Input: dimensioned drawing with shaded views. Units: mm. Origin: part minimum x, y, z. A direction names the side the tool comes from. Coordinates: 2 decimals unless noted, no trailing zeros. Loops run counter-clockwise (first coordinate to the right, second up) from the corner with the lowest first, then second, coordinate; pieces in that order, holes last.
Item 1: Section query B-B, the plane y = 1. Return the cut outline in (x, z).
Item 2: Reachability of the marked faces 1, 2, 3 and 4 from +Z, -Z, +X, -X, +Y, -Y: full face, straight path, thin tool, end or side. Return the list, or none.
Item 3: Line query: probe 1 along X at (y, z) = (5, 1.5); probe 2 along Z at (x, y) = (1.75, 4.25); probe 3 along Z at (x, y) = (5.75, 9.25). Output: solid intervals per line, ascending.
Item 4: Section query A-A, the plane z = 9.5. Return the cut outline in (x, y).
Item 5: Pin query (flat end, axial travel): pin 1 Ø1 at (x, z) = (3.5, 7.5) entering from +Y; pin 2 Ø1.5 at (x, z) = (2, 5.5) entering from -Y; pin 3 Ø1 at (y, z) = (1, 7) entering from -X. Return the tip coordinate at first contact, or that it passes through.
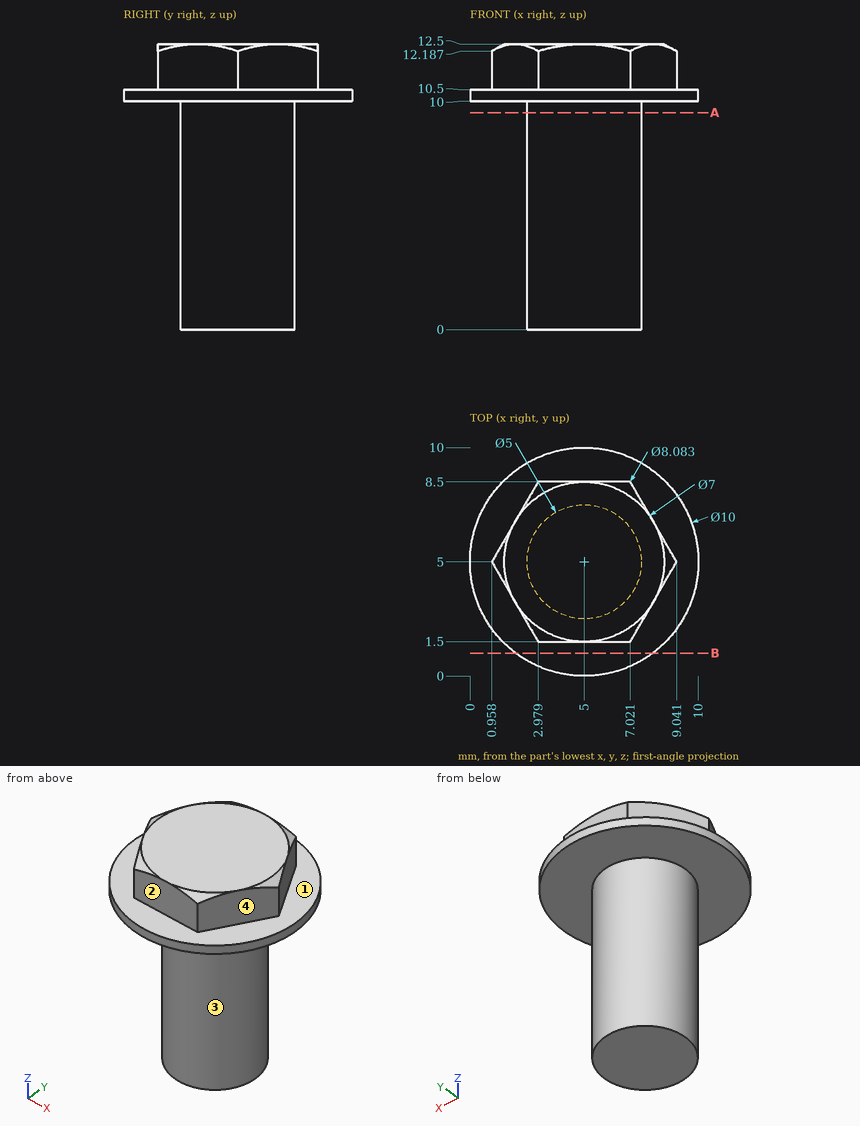
Verdict:
1. outline: (2, 10) - (8, 10) - (8, 10.5) - (2, 10.5) - close
2. face 1: +Z
2. face 2: +Z, +X, -X, -Y
2. face 3: -Z
2. face 4: +Z, +X, -Y
3. probe 1: x = 2.5 to 7.5
3. probe 2: z = 10 to 12.5
3. probe 3: z = 10 to 10.5
4. outline: circle Ø5 at (5, 5)
5. pin 1: stops at y = 7.29
5. pin 2: stops at y = 3.91
5. pin 3: passes through
